Design review of the part built by this model. Coordinates are the model's own, in mm. A direction names the side the tool comes from. Give positions to 0.01 mm unless a question says otherwise; leave off trailing zeros. Loops run counter-clockwise (first coordinate to the right, second up) from the corner with the lowest first, then second, coordinate; pieces in that order, holes last. Notation, with made-up numbers: (79, 54.25) -> (132, 54.25) arc R25 cw to (132, 82.25) -> close; hole circle Ø3 at (2, -40). An arc over 180 degrees is marked (long way). Use a Markdown table: item, result. Add a question column.
1. Add section A-A (y = 2.75). State the section outline as (x, z) points.
2. Add section B-B (z = 0). State the section outline as (x, y) points, and give its area (3 significant figures).
3. For pin 1 Ø1.5 at (x, z) = (0, 0) entering from +Y; pin 2 Ø3 at (y, z) = (-5, 0) entering from -X; pin 3 Ø2 at (x, z) = (-2.5, -1.5) entering from -Y, all flat-tipped, find the tip position at first contact; note any pin that passes through.
4. Add section C-C (y = -6). State the section outline as (x, z) points, and give its area (3 significant figures).
5. Draft analysis for pull direction X (two halves, no side actions). For faces 4 (the cylindrical face through (1.5, -8.04, -0.07)), 5 (the flat face through (-0.8, 3.5, -1.5)), 6 (the flat face through (0.76, 2.317, -1.293)), state which applies: pulls with the +X half, pulls with the -X half, needs draft (parallel to the pull), parting line crosses it, or undercut.
6. To check wall thickness, follow line 1 (Y direction, x = 0.5, z = -1.5); line 2 (Y direction, x = 3, z = 1); line 3 (X direction, y = 2.75, z = -1.25). State the ranges of each line that lie inside material, in increasing order.
7. For faces 1 (the cylindrical face through (0, -2, 2)), 2 (the flat face through (0, -11, 0)), 3 (the flat face through (0, 1.1, 0)), list the 3-axis set-ups (+Z, -Z, +X, -X, +Y, -Y) from which the entire face can be reached by the end or side of a thin tool; tool diameter is ignored.
```python
from build123d import *

# Parameters (mm, degrees)
FILLET1_R          = 0.3
CUT_EXTRUDE1_DEPTH = 2.4
CHAMFER1_SIZE      = 0.2


with BuildPart() as part:
    # Sketch1 → Revolve1 (revolve)
    with BuildSketch(Plane.XY):
        Polygon((0, 3.5), (-3.5, 3.5), (-3.5, 0), (-2, 0), (-2, -5), (-1.5, -5), (-1.5, -11), (0, -11), align=None)
    revolve(axis=Axis((0, 3.5, 0), (0, -1, 0)))

    # Fillet1
    fillet1_edges = [part.edges().sort_by_distance(p)[0] for p in [
        (3.5, 0, 0),
        (3.5, 3.5, 0),
    ]]
    fillet(fillet1_edges, radius=FILLET1_R)

    # Sketch2 → Cut-Extrude1 (cut)
    with BuildSketch(Plane(origin=(0, 3.5, 0), x_dir=(1, 0, 0), z_dir=(0, 1, 0))):
        Polygon((1.5, 0.866025404), (0, 1.732050808), (-1.5, 0.866025404), (-1.5, -0.866025404), (0, -1.732050808), (1.5, -0.866025404), align=None)
    extrude(amount=-CUT_EXTRUDE1_DEPTH, mode=Mode.SUBTRACT)

    # Chamfer1
    chamfer1_edges = [part.edges().sort_by_distance(p)[0] for p in [
        (2, -5, 0),
    ]]
    chamfer(chamfer1_edges, length=CHAMFER1_SIZE)


solid = part.part
```
Taken from the geometry:
| question | item | result |
|---|---|---|
| 1 | outline | circle Ø7 at (0, 0); hole (-1.5, -0.87) -> (0, -1.73) -> (1.5, -0.87) -> (1.5, 0.87) -> (0, 1.73) -> (-1.5, 0.87) -> close |
| 2 | outline | (-3.5, 0.3) arc R0.3 ccw to (-3.2, 0) -> (-2, 0) -> (-2, -4.8) -> (-1.8, -5) -> (-1.5, -5) -> (-1.5, -11) -> (1.5, -11) -> (1.5, -5) -> (1.8, -5) -> (2, -4.8) -> (2, 0) -> (3.2, 0) arc R0.3 ccw to (3.5, 0.3) -> (3.5, 3.2) arc R0.3 ccw to (3.2, 3.5) -> (1.5, 3.5) -> (1.5, 1.1) -> (-1.5, 1.1) -> (-1.5, 3.5) -> (-3.2, 3.5) arc R0.3 ccw to (-3.5, 3.2) -> close |
| 2 | area | 55.2 mm^2 |
| 3 | pin 1 | stops at y = 1.1 |
| 3 | pin 2 | stops at x = -2 |
| 3 | pin 3 | stops at y = -4.88 |
| 4 | outline | circle Ø3 at (0, 0) |
| 4 | area | 7.07 mm^2 |
| 5 | face 4 | parting line crosses it |
| 5 | face 5 | needs draft |
| 5 | face 6 | undercut |
| 6 | line 1 | y = -5 to 3.5 |
| 6 | line 2 | y = 0 to 3.5 |
| 6 | line 3 | x = -3.27 to -0.83, 0.83 to 3.27 |
| 7 | face 1 | -Y |
| 7 | face 2 | +Z, -Z, +X, -X, -Y |
| 7 | face 3 | +Y |
